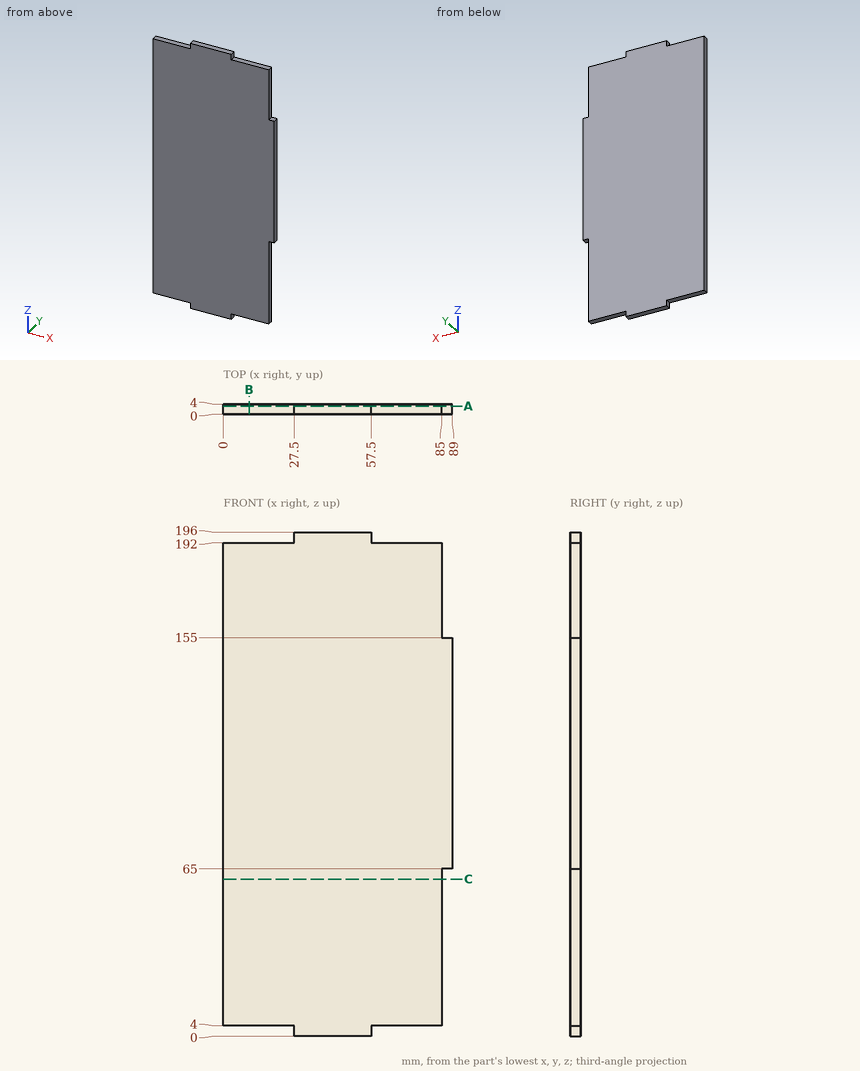
Here's the drawing with two shaded views (mm, measured from the low corner). I have some questions. Give positions to 0.01 mm unless a question says otherwise; leave off trailing zeros. Write each loop counter-clockwise with the first axis right and the second up, starting at its lowest first coordinate (ties: lowest second). Pieces come first, ordered by that corner, then holes. Notation, with made-up numbers: (66.5, -26.5) -> (72.5, -26.5) arc R17 ccw to (72.5, -12.5) -> close; hole circle Ø10 at (-19.5, -0.5). An arc over 180 degrees is marked (long way). One line per item, written item: value.
Q1. For P1, Ø8, axis at x = 44.5, z = 149, coming from the -Y side; P2, Ø1.2, axis at y = 1, z = 194.5, coming from the -X side; P3, Ø1.2, axis at x = 86.5, y = 2, coming from the -Z side; P4, Ø1.2, axis at x = 10.5, y = 1.5, coming from the +Z side, each with a flat end and sliding along its axis, tell me the tip position at first contact or that it passes through.
Results found:
P1: stops at y = 0
P2: stops at x = 27.5
P3: stops at z = 65
P4: stops at z = 192
Q2. Imagine slicing it at C-C on z = 61. Please give me the cut outline in (x, y).
Results found:
outline: (0, 0) -> (85, 0) -> (85, 4) -> (0, 4) -> close
Q3. Please list where these lines run through material, in increasing order: line 1 (X direction, y = 0.25, z = 63); line 2 (Z direction, x = 64, y = 0.9). Write a range as [from, to].
Results found:
line 1: x = [0, 85]
line 2: z = [4, 192]
Q4. Imagine slicing it at A-A on y = 3.2. Please give me the cut outline in (x, z), and give its area (3 significant figures).
Results found:
outline: (0, 4) -> (27.5, 4) -> (27.5, 0) -> (57.5, 0) -> (57.5, 4) -> (85, 4) -> (85, 65) -> (89, 65) -> (89, 155) -> (85, 155) -> (85, 192) -> (57.5, 192) -> (57.5, 196) -> (27.5, 196) -> (27.5, 192) -> (0, 192) -> close
area: 16,600 mm^2
Q5. Imagine slicing it at B-B on x = 10. Please give me the cut outline in (y, z), and give its area (3 significant figures).
Results found:
outline: (0, 4) -> (4, 4) -> (4, 192) -> (0, 192) -> close
area: 752 mm^2
